from build123d import *

# Parameters (mm, degrees)
SKETCH1_W           = 66
SKETCH1_H           = 49
BOSS_EXTRUDE1_DEPTH = 19
SHELL1_T            = -1.5
SKETCH2_W           = 6
SKETCH2_H           = 4.6
BOSS_EXTRUDE2_DEPTH = 17.5
FILLET1_R           = 1.5
SKETCH3_R           = 2.15
SKETCH3_R_2         = 1.45
BOSS_EXTRUDE3_DEPTH = 4.6
BOSS_EXTRUDE4_DEPTH = 0.5
FILLET2_R           = 4
FILLET3_R           = 2
BOSS_EXTRUDE5_REACH = 351.368
SKETCH5_R           = 3.5
FILLET4_R           = 2
SKETCH6_R           = 1
CUT_EXTRUDE1_DEPTH  = 350.367542449
FILLET5_R           = 1


with BuildPart() as part:
    # Sketch1 → Boss-Extrude1 (new body)
    with BuildSketch(Plane.XY.offset(30)):
        with Locations((105.809562907, 295.544660887)):
            Rectangle(SKETCH1_W, SKETCH1_H)
    extrude(amount=BOSS_EXTRUDE1_DEPTH)

    # Shell1
    shell1_openings = [part.faces().sort_by_distance(p)[0] for p in [
        (105.809562907, 295.544660887, 49),
    ]]
    offset(amount=SHELL1_T, openings=shell1_openings, kind=Kind.INTERSECTION)

    # Sketch2 → Boss-Extrude2 (add)
    with BuildSketch(Plane.XY.offset(31.5)):
        with Locations((90.011318394, 316.244660887)):
            Rectangle(SKETCH2_W, SKETCH2_H)
        with Locations((121.756668801, 316.244660887)):
            Rectangle(SKETCH2_W, SKETCH2_H)
    extrude(amount=BOSS_EXTRUDE2_DEPTH)

    # Fillet1
    fillet1_edges = [part.edges().sort_by_distance(p)[0] for p in [
        (74.309562907, 318.544660887, 40.25),
        (137.309562907, 318.544660887, 40.25),
        (72.809562907, 320.044660887, 39.5),
        (138.809562907, 320.044660887, 39.5),
    ]]
    fillet(fillet1_edges, radius=FILLET1_R)

    # Sketch3 → Boss-Extrude3 (add)
    # profile 1 of 4: a face of its own
    with BuildSketch(Plane.XY.offset(31.5)):
        with Locations((90.939840403, 307.111410879)):
            Circle(SKETCH3_R)
        with Locations((90.939840403, 307.111410879)):
            Circle(SKETCH3_R_2, mode=Mode.SUBTRACT)
    # profile 2 of 4: a face of its own
    with BuildSketch(Plane.XY.offset(31.5)):
        with Locations((120.939840403, 307.111410879)):
            Circle(SKETCH3_R)
        with Locations((120.939840403, 307.111410879)):
            Circle(SKETCH3_R_2, mode=Mode.SUBTRACT)
    # profile 3 of 4: a face of its own
    with BuildSketch(Plane.XY.offset(31.5)):
        with Locations((120.939840403, 292.111410879)):
            Circle(SKETCH3_R)
        with Locations((120.939840403, 292.111410879)):
            Circle(SKETCH3_R_2, mode=Mode.SUBTRACT)
    # profile 4 of 4: a face of its own
    with BuildSketch(Plane.XY.offset(31.5)):
        with Locations((90.939840403, 292.111410879)):
            Circle(SKETCH3_R)
        with Locations((90.939840403, 292.111410879)):
            Circle(SKETCH3_R_2, mode=Mode.SUBTRACT)
    extrude(amount=BOSS_EXTRUDE3_DEPTH)

    # Sketch4 → Boss-Extrude4 (add, symmetric)
    with BuildSketch(Plane(origin=(0, 284, 0), x_dir=(1, 0, 0), z_dir=(0, 1, 0))):
        Polygon((72.809562907, -47.615589413), (78.809562907, -47.615589413), (78.809562907, -37.615589413), (132.809562907, -37.615589413), (132.809562907, -47.615589413), (138.809562907, -47.615589413), (138.809562907, -30), (72.809562907, -30), align=None)
    extrude(amount=BOSS_EXTRUDE4_DEPTH, both=True)

    # Fillet2
    fillet2_edges = [part.edges().sort_by_distance(p)[0] for p in [
        (78.809562907, 284, 47.615589413),
        (132.809562907, 284, 47.615589413),
    ]]
    fillet(fillet2_edges, radius=FILLET2_R)

    # Fillet3
    fillet3_edges = [part.edges().sort_by_distance(p)[0] for p in [
        (78.809562907, 284, 37.615589413),
        (132.809562907, 284, 37.615589413),
    ]]
    fillet(fillet3_edges, radius=FILLET3_R)

    # Boss-Extrude5: up to this face of the body (flat: up to its plane)
    boss_extrude5_end = Plane(part.part.faces().sort_by_distance((105.809562907, 295.537442811, 30))[0])
    # Sketch5 → Boss-Extrude5 (add, up to the picked face)
    with BuildSketch(Plane.XY.offset(49), mode=Mode.PRIVATE) as boss_extrude5_sk1:
        with Locations((76.56102911, 270.299359986)):
            Circle(SKETCH5_R)
    boss_extrude5_tool1 = split(extrude(boss_extrude5_sk1.sketch, amount=-BOSS_EXTRUDE5_REACH, mode=Mode.PRIVATE), bisect_by=boss_extrude5_end, keep=Keep.BOTH, mode=Mode.PRIVATE)
    # Sketch5 → Boss-Extrude5 (add, up to the picked face)
    with BuildSketch(Plane.XY.offset(49), mode=Mode.PRIVATE) as boss_extrude5_sk2:
        with Locations((135, 270)):
            Circle(SKETCH5_R)
    boss_extrude5_tool2 = split(extrude(boss_extrude5_sk2.sketch, amount=-BOSS_EXTRUDE5_REACH, mode=Mode.PRIVATE), bisect_by=boss_extrude5_end, keep=Keep.BOTH, mode=Mode.PRIVATE)
    add(boss_extrude5_tool1.solids().sort_by(Axis((76.561029, 270.29936, 49), (0, 0, -1)))[0])
    add(boss_extrude5_tool2.solids().sort_by(Axis((135, 270, 49), (0, 0, -1)))[0])

    # Fillet4
    fillet4_edges = [part.edges().sort_by_distance(p)[0] for p in [
        (79.980755206, 271.044660887, 39.5),
        (131.659538411, 271.044660887, 39.5),
        (87.011318394, 313.944660887, 40.25),
        (93.011318394, 313.944660887, 40.25),
        (118.756668801, 313.944660887, 40.25),
        (124.756668801, 313.944660887, 40.25),
    ]]
    fillet(fillet4_edges, radius=FILLET4_R)

    # Sketch6 → Cut-Extrude1 (cut, through all)
    with BuildSketch(Plane.XY.offset(49)):
        with Locations((89.892121314, 316.968054702)):
            Circle(SKETCH6_R)
        with Locations((122.022521406, 316.968054702)):
            Circle(SKETCH6_R)
        with Locations((75.978849521, 269.963322555)):
            Circle(SKETCH6_R)
        with Locations((135.943985107, 269.963322555)):
            Circle(SKETCH6_R)
    extrude(amount=-CUT_EXTRUDE1_DEPTH, mode=Mode.SUBTRACT)

    # Fillet5
    # the kernel refuses this fillet: 1 mm, written as the material it takes off along each edge
    with BuildSketch(Plane(origin=(72.809562907, 271.044660887, 28.140180255), x_dir=(1, 0, 0), z_dir=(0, 0, 1))) as fillet5_piece_1:
        with BuildLine():
            CenterArc((1, 0.743927898), FILLET5_R, 180, 48.067095939)
            Line((0, 0.743927898), (-0.02, 0.743927898))
            Line((-0.02, 0.743927898), (-0.02, 0))
            Line((-0.02, 0), (0, -0.02))
            ThreePointArc((0, -0.02), (0.165870054, -0.02), (0.31837491, -0.014878558))
            Line((0.31837491, -0.014878558), (0.331740108, 0))
        make_face()
    extrude(amount=22.719639489, mode=Mode.SUBTRACT)
    with BuildSketch(Plane(origin=(138.809562907, 271.044660887, 27.881411748), x_dir=(-1, 0, 0), z_dir=(0, 0, 1))) as fillet5_piece_2:
        with BuildLine():
            CenterArc((1, -0.847435301), FILLET5_R, 122.066195324, 57.933804676)
            Line((0, -0.847435301), (-0.02, -0.847435301))
            Line((-0.02, -0.847435301), (-0.02, 0))
            Line((-0.02, 0), (0, 0.02))
            ThreePointArc((0, 0.02), (0.234550659, 0.02), (0.458483344, 0.016948706))
            Line((0.458483344, 0.016948706), (0.469101317, 0))
        make_face()
    extrude(amount=23.237176503, mode=Mode.SUBTRACT)


solid = part.part
Design review of the part built by this model. Coordinates are the model's own, in mm. A direction names the side the tool comes from. Round coordinates to 2 decimals unless told otherwise and drop trailing zeros. Order: outer loops, then holes, each group sorted by start corner. A loop starts at its lowest first (then second) coordinate and runs counter-clockwise, first axis right, second up. Notation, with made-up numbers: M 77,-1.75 L 91,-1.75 A10 cw 91,16.25 Z; hole C -33,62 d10. An arc over 180 degrees is marked long. Answer as CSV lines item,"result". Start each with the question number.
1) Tool access review of faces 1 (the face through (80.688, 270.623, 39.633)), 2 (the face through (119, 307, 36.1)), 3 (the face through (121.89, 317.96, 39.63)): name each direction out of +Z, -Z, +X, -X, +Y, -Y from which nothing blocks a thin tool from reaching the whole face with its end or side.
2) For pin 1 Ø8 at (x, z) = (113, 36.5) entering from -Y; pin 2 Ø3.5 at (x, z) = (129.5, 44) entering from -Y; pin 3 Ø2 at (x, y) = (120.5, 305.5) entering from +Z, all flat-tipped, find the tip position at first contact; note any pin that passes through.
3) Add section A-A (x = 125.5). Give the boundary of the cut face in (y, z), then the cut area to 3 significant figures.
4) Add section B-B (z = 40.75). Give the number of separate pieces and of enclosed holes in the cut face, then the cut area to 3 significant figures.
5) The part is to be moulded in two halves that separate along X. For faces 4 (the face through (119, 292, 36.1)), 5 (the face through (73.237, 319.594, 39.633)), 6 (the face through (103, 272, 49)), say which applies: +X half, -X half, draft (parallel to the pull), parting line (faces both ways), or undercut.
6) Wall thickness on line 1 along Y through (x, z) = (127, 32.25); line 2 along Y through (x, z) = (90, 44); line 3 along X through (y, z) = (317, 41.5): over which ranges is each line inside the solid? List them lowest first. Write a range as [from, to].
Resolved:
1,face 1,"+Z, -Z, -Y"
1,face 2,"+Z"
1,face 3,"+Z, -Z"
2,pin 1,"y = 271.04"
2,pin 2,"y = 270.15"
2,pin 3,"z = 36.1"
3,outline,"M 271.04,30 L 320.04,30 L 320.04,49 L 318.54,49 L 318.54,31.5 L 284.5,31.5 L 284.5,37.62 L 283.5,37.62 L 283.5,31.5 L 272.54,31.5 L 272.54,49 L 271.04,49 Z"
3,area,"132 mm^2"
4,separate pieces,"1"
4,enclosed holes,"5"
4,area,"444 mm^2"
5,face 4,"undercut"
5,face 5,"-X half"
5,face 6,"draft"
6,line 1,"[271.04, 272.54], [283.5, 284.5], [318.54, 320.04]"
6,line 2,"[271.04, 272.54], [313.94, 315.97], [317.96, 320.04]"
6,line 3,"[72.81, 74.31], [87.01, 88.89], [90.89, 93.01], [118.76, 121.02], [123.02, 124.76], [137.31, 138.81]"
